Drawing for the job (mm, zero at the part's lowest x, y, z). A direction names the side the tool comes from. Give positions to 0.01 mm unless a question says otherwise; leave off trailing zeros. Order: outer loops, then holes, each group sorted by start corner. A loop starts at its lowest first (then second) coordinate and runs counter-clockwise, first axis right, second up. Notation, with made-up numbers: (-27.5, 63.25) -> (4.5, 63.25) arc R28 cw to (4.5, 85.25) -> close; hole circle Ø9 at (1, 85). An arc over 180 degrees is marked (long way). One line per item, written item: value. Start each with the question number.
(1) Which spindle directions (+Z, -Z, +X, -X, +Y, -Y) get a long thin tool onto all of the face, cutting with end or side? Do the marked faces 5 and 6. Say none if no direction does.
(2) Saw through at A-A on x = 31.75. Give the cut face in (y, z).
(3) Probe line 1 (Z direction, x = 43, y = 1); line 2 (X direction, y = 27, z = 5.5). List the from-to ranges inside material, lowest first.
(4) Saw through at B-B on y = 4. Count the separate pieces of the cut face and the enclosed holes in it, plus the area to 3 significant figures.
(5) Saw through at C-C on z = 8.5. Give the cut face in (x, y).
(6) Two-plate mould, pull along Z, no slides. Class the marked faces 1, 2, 3 and 4: +Z half, -Z half, draft (parallel to the pull), parting line (faces both ways), or undercut.
(7) Pin check, flat tips, straight feed: pin 1 (10 mm diameter, centred on x = 12, y = 15, fed in from +Z); pin 2 (20.5 mm diameter, centred on x = 21, z = 16, fed in from +Y); pin 3 (12.5 mm diameter, centred on y = 28.5, z = 28.5, fed in from +X). Stop position of each tip, or through.
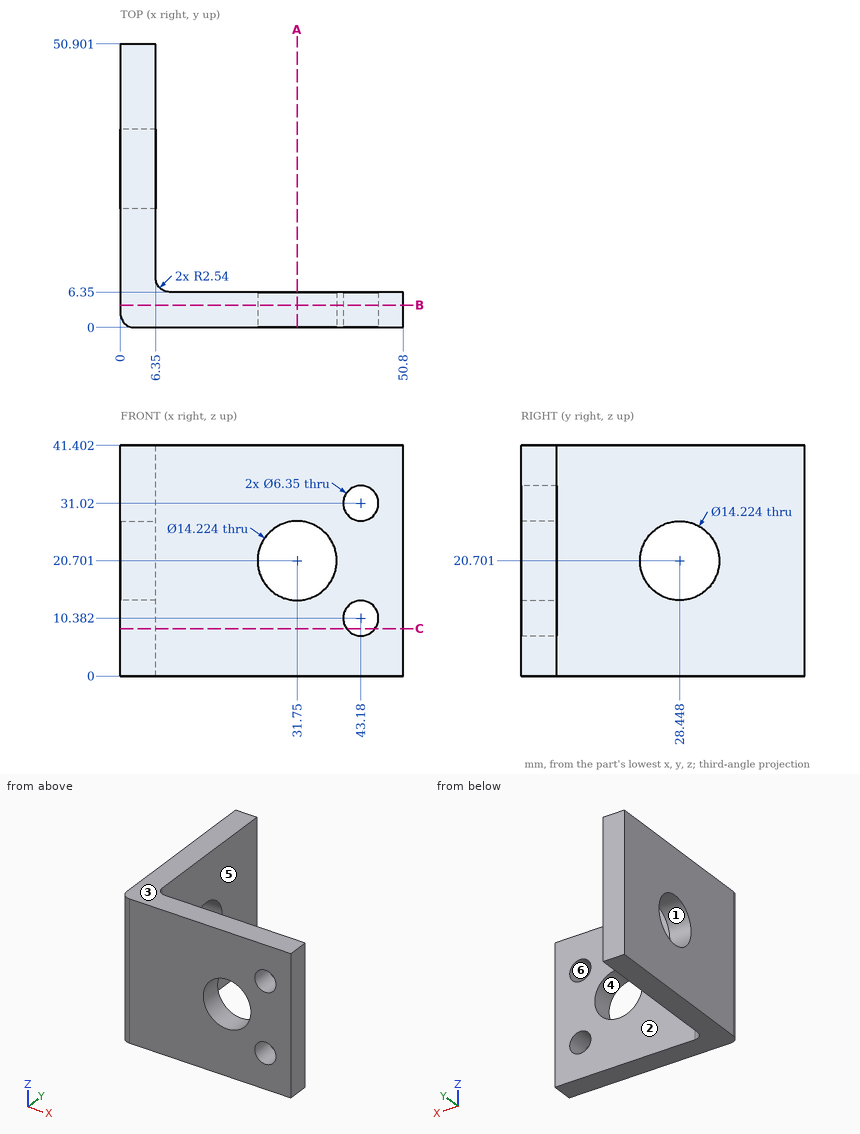
Results below:
1. face 5: +Z, -Z, +X, +Y
1. face 6: +Y, -Y
2. outline: (0, 0) -> (6.35, 0) -> (6.35, 13.59) -> (0, 13.59) -> close; (0, 27.81) -> (6.35, 27.81) -> (6.35, 41.4) -> (0, 41.4) -> close
3. line 1: z = 0 to 7.21, 13.55 to 27.85, 34.19 to 41.4
3. line 2: x = 0 to 6.35
4. separate pieces: 1
4. enclosed holes: 3
4. area: 1,880 mm²
5. outline: (0, 2.54) arc R2.54 ccw to (2.54, 0) -> (40.62, 0) -> (40.62, 6.35) -> (8.89, 6.35) arc R2.54 cw to (6.35, 8.89) -> (6.35, 50.9) -> (0, 50.9) -> close; (45.74, 0) -> (50.8, 0) -> (50.8, 6.35) -> (45.74, 6.35) -> close
6. face 1: undercut
6. face 2: draft
6. face 3: +Z half
6. face 4: undercut
7. pin 1: passes through
7. pin 2: stops at y = 6.35
7. pin 3: stops at x = 6.35
